```python
from build123d import *
from build123d.topology import SkipClean

# Parameters (mm, degrees)
BOSS_EXTRUDE1_DEPTH   = 10
BOSS_EXTRUDE1_2_DEPTH = 10
BOSS_EXTRUDE1_3_DEPTH = 10
BOSS_EXTRUDE1_4_DEPTH = 10
SKETCH3_R             = 50
BOSS_EXTRUDE2_DEPTH   = 10


with BuildPart() as part:
    # Sketch2 → Boss-Extrude1 (new body)
    with BuildSketch(Plane.XY):
        with BuildLine():
            Line((4.12040185, 49.82993366), (4.12040185, 5.879436141))
            Line((4.12040185, 5.879436141), (49.653119043, 5.879436141))
            ThreePointArc((49.653119043, 5.879436141), (34.724767031, 35.974860036), (4.12040185, 49.82993366))
        make_face()
    extrude(amount=BOSS_EXTRUDE1_DEPTH)



with BuildPart() as body_2:
    # Sketch2 → Boss-Extrude1 2 (new body)
    with BuildSketch(Plane.XY):
        with BuildLine():
            Line((-5.87959815, 49.653099859), (-5.87959815, 5.879436141))
            Line((-5.87959815, 5.879436141), (-49.653119043, 5.879436141))
            ThreePointArc((-49.653119043, 5.879436141), (-35.355396738, 35.35528138), (-5.87959815, 49.653099859))
        make_face()
    extrude(amount=BOSS_EXTRUDE1_2_DEPTH)


with BuildPart() as body_3:
    # Sketch2 → Boss-Extrude1 3 (new body)
    with BuildSketch(Plane.XY):
        with BuildLine():
            Line((-49.829920264, -4.120563859), (-5.87959815, -4.120563859))
            Line((-5.87959815, -4.120563859), (-5.87959815, -49.653099859))
            ThreePointArc((-5.87959815, -49.653099859), (-35.974860237, -34.724766823), (-49.829920264, -4.120563859))
        make_face()
    extrude(amount=BOSS_EXTRUDE1_3_DEPTH)


with BuildPart() as body_4:
    # Sketch2 → Boss-Extrude1 4 (new body)
    with BuildSketch(Plane.XY):
        with BuildLine():
            Line((4.12040185, -4.120563859), (4.12040185, -49.82993366))
            ThreePointArc((4.12040185, -49.82993366), (35.355281585, -35.355396534), (49.829920264, -4.120563859))
            Line((49.829920264, -4.120563859), (4.12040185, -4.120563859))
        make_face()
    extrude(amount=BOSS_EXTRUDE1_4_DEPTH)


with BuildPart() as part_1:
    with SkipClean():  # the faces are left unmerged after this step: merging them gives an invalid solid
        add(part.part)

        add(body_2.part)  # Boss-Extrude2 merges body 2

        add(body_3.part)  # Boss-Extrude2 merges body 3

        add(body_4.part)  # Boss-Extrude2 merges body 4
        # Sketch3 → Boss-Extrude2 (add)
        with BuildSketch(Plane.XY.offset(10)):
            with Locations(Location((0, 0, 0), (0, 0, 184.727179566))):
                Circle(SKETCH3_R)
        extrude(amount=BOSS_EXTRUDE2_DEPTH)


solid = part_1.part
```
Read the model definition and answer for the solid it produces. Units are mm, in the model's axes. A direction names the side the tool comes from. Coordinates: 2 decimals unless noted, no trailing zeros. Order: outer loops, then holes, each group sorted by start corner. A loop starts at its lowest first (then second) coordinate and runs counter-clockwise, first axis right, second up. Notation, with made-up numbers: (67.5, -22.75) - (84.5, -22.75) arc R22 cw to (84.5, -1.75) - close; hole circle Ø1 at (-33, 65.25). An arc over 180 degrees is marked (long way). Answer as a JSON object with one key per item and string values. Group by question number.
Item 1: The mould has two halves that part along X. Classify faces 1 (the face through (4.12, 28, 5)), 2 (the face through (22, 23, 0)): +X half, -X half, draft (parallel to the pull), parting line (faces both ways), or undercut.
Item 2: Consider probe 1 along Y at (x, z) = (-6, 2.75); probe 2 along Y at (x, z) = (-32, 5); probe 3 along X at (y, z) = (-6.5, 7). Determine where each line is inside the solid, lowest interval first. Write a range as from..to.
Item 3: A tool of negligible diameter and unlimited length cuts with its end or side. For faces 3 (the face through (-5.88, 28, 5)), 4 (the face through (22, -22, 0)), 5 (the face through (27, 5.879, 5)), from which of +Z, -Z, +X, -X, +Y, -Y can it reach the whole face along a straight path? Write none if from no direction.
Item 4: Section D-D (z = 18) is taken. Give the vertices of the cut face in (x, y).
Item 5: Section A-A (z = 7) is taken. Give the vertices of the cut face in (x, y), plus the area to 3 significant figures.
Item 6: Flat-ended cylindrical pins translate along their axes: P1, Ø3, axis at y = -39, z = 13, coming from the -X side; P2, Ø3, axis at y = -32, z = 5.5, coming from the -X side; P3, Ø2, axis at y = 31.5, z = 14.5, coming from the +X side. Find the tip coordinate at first contact, or state that the pin passes through.
Item 7: Section B-B (y = 42) is taken. Give the vertices of the cut face in (x, z).
Item 8: Section C-C (x = -14) is taken. Give the vertices of the cut face in (y, z), plus the area to 3 significant figures.
Results are:
{
 "1": {"face 1": "undercut", "face 2": "draft"},
 "2": {"probe 1": "y = -49.64..-4.12, 5.88..49.64", "probe 2": "y = -38.42..-4.12, 5.88..38.42", "probe 3": "x = -49.58..-5.88, 4.12..49.58"},
 "3": {"face 3": "-Z, +Y, -Y", "face 4": "-Z, +X, -X, +Y, -Y", "face 5": "-Z, +X, -X"},
 "4": {"outline": "circle Ø100 at (0, 0)"},
 "5": {"outline": "(-49.83, -4.12) arc R50 ccw to (-5.88, -49.65) - (-5.88, -4.12) - close; (-49.65, 5.88) - (-5.88, 5.88) - (-5.88, 49.65) arc R50 ccw to start; (4.12, -49.83) arc R50 ccw to (49.83, -4.12) - (4.12, -4.12) - close; (4.12, 5.88) - (49.65, 5.88) arc R50 ccw to (4.12, 49.83) - close", "area": "5,960 mm^2"},
 "6": {"P1": "stops at x = -33.07", "P2": "stops at x = -39.62", "P3": "stops at x = 39.62"},
 "7": {"outline": "(-27.13, 0) - (-5.88, 0) - (-5.88, 10) - (4.12, 10) - (4.12, 0) - (27.13, 0) - (27.13, 20) - (-27.13, 20) - close"},
 "8": {"outline": "(-48, 0) - (-4.12, 0) - (-4.12, 10) - (5.88, 10) - (5.88, 0) - (48, 0) - (48, 20) - (-48, 20) - close", "area": "1,820 mm^2"}
}
